from build123d import *

# Parameters (mm, degrees)
PAD029_DEPTH         = 50
PAD029_DEPTH_BACK    = 40
POCKET025_DEPTH      = 37
POCKET025_DEPTH_BACK = 100
FILLET018_R          = 2
SKETCH057_R          = 2.3
POCKET026_DEPTH      = 15
CHAMFER013_SIZE      = 1


with BuildPart() as part:
    # Sketch055 → Pad029 (new body, two sides)
    with BuildSketch(Plane.YZ) as pad029_sk:
        with BuildLine():
            Line((0, 19), (0, -19))
            Line((0, -19), (28.9586804597, -60.3572817765))
            ThreePointArc((40, -22.0491502813), (28.9668360053, -39.6143804936), (28.9586804597, -60.3572817765))
            Line((40, 22.0491502813), (40, -22.0491502813))
            ThreePointArc((28.9586804597, 60.3572817765), (28.9668360053, 39.6143804936), (40, 22.0491502813))
            Line((0, 19), (28.9586804597, 60.3572817765))
        make_face()
    extrude(amount=PAD029_DEPTH)
    extrude(pad029_sk.sketch, amount=-PAD029_DEPTH_BACK)

    # Sketch056 → Pocket025 (cut, two sides)
    with BuildSketch(Plane.YZ) as pocket025_sk:
        with BuildLine():
            ThreePointArc((28.9586804597, 60.3572817765), (27.6278296398, 46.9063156967), (31.1523619549, 33.8572803169))
            ThreePointArc((31.1523619549, 33.8572803169), (32.3065923695, 31.6317911188), (33.6069416835, 29.4883962222))
            Line((33.6069416835, 29.4883962222), (0, 13.4604701885))
            Line((0, 13.4604701885), (0, 19))
            Line((0, 19), (28.9586804597, 60.3572817765))
        make_face()
    extrude(amount=-POCKET025_DEPTH, mode=Mode.SUBTRACT)
    extrude(pocket025_sk.sketch, amount=POCKET025_DEPTH_BACK, mode=Mode.SUBTRACT)

    # Fillet018
    fillet018_edges = [part.edges().sort_by_distance(p)[0] for p in [
        (-38.5, 28.95868, 60.357282),
    ]]
    fillet(fillet018_edges, radius=FILLET018_R)

    # Sketch057 → Pocket026 (cut)
    with BuildSketch(Plane(origin=(0, -5.2300130023, 10.9661562951), x_dir=(1, 0, 0), z_dir=(0, -0.4304725249, 0.9026036812))):
        with Locations((45, 33.027693654)):
            Circle(SKETCH057_R)
    extrude(amount=-POCKET026_DEPTH, mode=Mode.SUBTRACT)

    # Chamfer013
    chamfer013_edges = [part.edges().sort_by_distance(p)[0] for p in [
        (42.7, 24.580905, 25.183671),
    ]]
    chamfer(chamfer013_edges, length=CHAMFER013_SIZE)


with BuildPart() as part_1:
    # Body029 placement: moved
    add(part.part.moved(Location((0, 10, 0))))


solid = part_1.part
The listing builds one solid part. Answer for the finished solid, in the listing's coordinates (mm). A direction names the side the tool comes from. Round coordinates to 2 decimals unless told otherwise and drop trailing zeros. Write each loop counter-clockwise with the first axis right and the second up, starting at its lowest first coordinate (ties: lowest second). Pieces come first, ordered by that corner, then holes. Notation, with made-up numbers: (35.5, -14) - (57.5, -14) arc R29 ccw to (57.5, 10) - close; hole circle Ø10 at (-39, -37). An arc over 180 degrees is marked (long way). Use one line per item in the form item = value. Start each with the question number.
Item 1: A cutting plane is placed at D-D (z = -27.5). Write down the section's boundary in (x, y).
Item 2: A cutting plane is placed at B-B (y = 26). Write down the section's boundary in (x, z).
Item 3: A cutting plane is placed at C-C (z = -40). Write down the section's boundary in (x, y), plus the area to 3 significant figures.
Item 4: A tool of negligible diameter and unlimited length cuts with its end or side. For faces 1 (the flat face through (44.97, 41.07, 11.66)), 2 (the cylindrical face through (5.63, 39.05, -39.33)), 3 (the flat face through (7.109, 27.039, 21.587)), from which of +Z, -Z, +X, -X, +Y, -Y can it reach the whole face along a straight path? Write none if from no direction.
Item 5: A cutting plane is placed at A-A (x = 15). Write down the section's boundary in (y, z).
Item 6: Find the intervals of material crossed by line 1 (X direction, y = 33.5, z = 24.5); line 2 (Z direction, x = -17, y = 46); line 3 (X direction, y = 35, z = 32.5), in increasing order. Write a range as [from, to].
Item 7: Determine the mould class of faces 4 (the flat face through (6, 10, 0)), 5 (the flat face through (-37, 27, 34)), 6 (the cylindrical face through (44.7, 40.04, 19.03)) for opening direction X: +X half, -X half, draft (parallel to the pull), parting line (faces both ways), or undercut.
Item 8: A flat-ended cylindrical pin translates along its axis: pin 1 Ø5 at (x, y) = (5.5, 26.5) entering from -Z. Find the tip coordinate at first contact, or state that the pin passes through.
The answers:
q1.outline = (-40, 15.95) - (50, 15.95) - (50, 45) - (-40, 45) - close
q2.outline = (-40, -41.85) - (50, -41.85) - (50, 21.09) - (-37, 21.09) - (-37, 41.85) - (-40, 41.85) - close
q3.outline = (-40, 24.7) - (50, 24.7) - (50, 38.86) - (-40, 38.86) - close
q3.area = 1,270 mm^2
q4.face_1 = none
q4.face_2 = +X, -X, +Y
q4.face_3 = +Z, +X, -Y
q5.outline = (10, -19) - (38.96, -60.36) arc R37.5 cw to (50, -22.05) - (50, 22.05) arc R37.5 cw to (43.61, 29.49) - (10, 13.46) - close
q6.line_1 = [-40, 42.12], [47.88, 50]
q6.line_2 = [-26.23, 26.23]
q6.line_3 = [-40, -37]
q7.face_4 = draft
q7.face_5 = +X half
q7.face_6 = undercut
q8.pin_1 = -46.13
